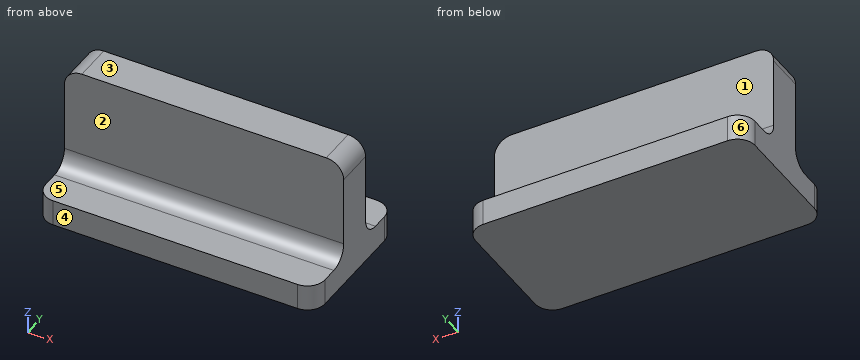
```python
from build123d import *

# Parameters (mm, degrees)
SKETCH1_W           = 50.8
SKETCH1_H           = 25.4
BOSS_EXTRUDE1_DEPTH = 4.7625
SKETCH2_W           = 50.8
SKETCH2_H           = 7
BOSS_EXTRUDE2_DEPTH = 19.05
FILLET1_R           = 3.175


with BuildPart() as part:
    # Sketch1 → Boss-Extrude1 (new body)
    with BuildSketch(Plane.XY):
        Rectangle(SKETCH1_W, SKETCH1_H)
    extrude(amount=BOSS_EXTRUDE1_DEPTH)

    # Sketch2 → Boss-Extrude2 (add)
    with BuildSketch(Plane.XY.offset(4.7625)):
        Rectangle(SKETCH2_W, SKETCH2_H)
    extrude(amount=BOSS_EXTRUDE2_DEPTH)

    # Fillet1
    fillet1_edges = [part.edges().sort_by_distance(p)[0] for p in [
        (0, 3.5, 4.7625),
        (0, -3.5, 4.7625),
        (25.4, 0, 23.8125),
        (-25.4, 0, 23.8125),
        (25.4, -12.7, 2.38125),
        (-25.4, -12.7, 2.38125),
        (-25.4, 12.7, 2.38125),
        (25.4, 12.7, 2.38125),
    ]]
    fillet(fillet1_edges, radius=FILLET1_R)


solid = part.part
```
Build history of the part. All positions in model axes, mm. Face numbers are marked on the shaded views. A direction names the side the tool comes from. Give positions to 0.01 mm unless a question says otherwise; leave off trailing zeros. Loops run counter-clockwise (first coordinate to the right, second up) from the corner with the lowest first, then second, coordinate; pieces in that order, holes last. Notation, with made-up numbers: (9.25, 84) -> (63.25, 84) arc R17 ccw to (63.25, 93) -> close; hole circle Ø10 at (2.5, 51.5). An arc over 180 degrees is marked (long way). One line per question, with ' | ' between items. Start each with the question number.
1) 3-axis set-ups, long thin cutter, end or side, ignore diameter. For the marked faces 1, 2 and 3: which of +Z, -Z, +X, -X, +Y, -Y reach the whole face in a straight line?
2) Pin check, flat tips, straight feed: pin 1 (5 mm diameter, centred on x = 12, z = 19.5, fed in from -Y); pin 2 (4 mm diameter, centred on x = -11, z = 9.5, fed in from +Y); pin 3 (1.5 mm diameter, centred on x = -8.5, z = 6, fed in from +Y); pin 4 (12 mm diameter, centred on x = 16.5, y = -8, fed in from -Z). Stop position of each tip, or through.
3) Two-plate mould, pull along Y, no slides. Class the marked faces 4, 5 and 6: released by +Y, released by -Y, zero draft, split by the parting line, or undercut.
4) Cut at B-B (z = 10.75). Give the cut face in (x, y), plus the area to 3 significant figures.
5) Probe L1, parallel to Y at x = 22.5, z = 15; L2, parallel to Z at x = -19.5, y = -8.5; L3, parallel to Z at x = 15.5, y = 5.5. List the from-to ranges inside material, lowest first.
6) Cut at C-C (y = -8.25). Give the cut face in (x, z).
Return value:
1) face 1: +Z, +X, -X, +Y | face 2: +Z, +X, -X, -Y | face 3: +Z, +X, -X, +Y, -Y
2) pin 1: y = -3.5 | pin 2: y = 3.53 | pin 3: y = 4.98 | pin 4: z = 0
3) face 4: released by -Y | face 5: zero draft | face 6: released by +Y
4) outline: (-25.4, -3.5) -> (25.4, -3.5) -> (25.4, 3.5) -> (-25.4, 3.5) -> close | area: 356 mm^2
5) L1: -3.5 to 3.5 | L2: 0 to 4.76 | L3: 0 to 4.99
6) outline: (-25.4, 0) -> (25.4, 0) -> (25.4, 4.76) -> (-25.4, 4.76) -> close
